Could you check a few things on this model? Use its own coordinates, in mm. Give positions to 0.01 mm unless a question says otherwise; leave off trailing zeros. Write each loop counter-clockwise with the first axis right and the second up, starting at its lowest first coordinate (ties: lowest second). Pieces come first, ordered by that corner, then holes. Notation, with made-up numbers: (-38.5, 48) -> (-18.5, 48) arc R21 ccw to (-18.5, 69) -> close; hole circle Ø2 at (-1.75, -17.5). An arc over 180 degrees is marked (long way). One line per question, with ' | ' between items.
from build123d import *

# Parameters (mm, degrees)
MODEL_R                 = 1.5
SALIENTE_EXTRUIR1_DEPTH = 3


with BuildPart() as part:
    # Model → Saliente-Extruir1 (new body)
    with BuildSketch(Plane.XY):
        with BuildLine():
            Line((-105.943383637, 101.056539338), (-105.943383637, 56.056539338))
            ThreePointArc((-105.943383637, 56.056539338), (-104.625364152, 52.874558823), (-101.443383637, 51.556539338))
            Line((-101.443383637, 51.556539338), (-56.443383637, 51.556539338))
            ThreePointArc((-56.443383637, 51.556539338), (-54.721308191, 51.899081442), (-53.261403122, 52.874558823))
            Line((-53.261403122, 52.874558823), (-104.625364152, 104.238519853))
            ThreePointArc((-104.625364152, 104.238519853), (-105.600841533, 102.778614784), (-105.943383637, 101.056539338))
        make_face()
        with Locations((-101.443383637, 92.056539338)):
            Circle(MODEL_R, mode=Mode.SUBTRACT)
        with Locations((-101.443383637, 83.056539338)):
            Circle(MODEL_R, mode=Mode.SUBTRACT)
        with Locations((-92.443383637, 83.056539338)):
            Circle(MODEL_R, mode=Mode.SUBTRACT)
        with Locations((-101.443383637, 74.056539338)):
            Circle(MODEL_R, mode=Mode.SUBTRACT)
        with Locations((-92.443383637, 74.056539338)):
            Circle(MODEL_R, mode=Mode.SUBTRACT)
        with Locations((-83.443383637, 74.056539338)):
            Circle(MODEL_R, mode=Mode.SUBTRACT)
        with Locations((-101.443383637, 65.056539338)):
            Circle(MODEL_R, mode=Mode.SUBTRACT)
        with Locations((-92.443383637, 65.056539338)):
            Circle(MODEL_R, mode=Mode.SUBTRACT)
        with Locations((-83.443383637, 65.056539338)):
            Circle(MODEL_R, mode=Mode.SUBTRACT)
        with Locations((-74.443383637, 65.056539338)):
            Circle(MODEL_R, mode=Mode.SUBTRACT)
        with Locations((-101.443383637, 56.056539338)):
            Circle(MODEL_R, mode=Mode.SUBTRACT)
        with Locations((-92.443383637, 56.056539338)):
            Circle(MODEL_R, mode=Mode.SUBTRACT)
        with Locations((-83.443383637, 56.056539338)):
            Circle(MODEL_R, mode=Mode.SUBTRACT)
        with Locations((-74.443383637, 56.056539338)):
            Circle(MODEL_R, mode=Mode.SUBTRACT)
        with Locations((-65.443383637, 56.056539338)):
            Circle(MODEL_R, mode=Mode.SUBTRACT)
    extrude(amount=SALIENTE_EXTRUIR1_DEPTH)


solid = part.part
Q1. If I drill on line 1 along X through (y, z) = (55, 2.15); line 2 along Y through (x, z) = (-73.5, 0.25); line 3 along Y through (x, z) = (-100.5, 2.9), over which ranges is the centre line in solid material (lowest first)?
Answer below:
line 1: x = -105.82 to -102.51, -100.38 to -93.51, -91.38 to -84.51, -82.38 to -75.51, -73.38 to -66.51, -64.38 to -55.39 | line 2: y = 51.56 to 54.89, 57.22 to 63.89, 66.22 to 73.11 | line 3: y = 51.56 to 54.89, 57.22 to 63.89, 66.22 to 72.89, 75.22 to 81.89, 84.22 to 90.89, 93.22 to 100.11
Q2. Imagine slicing it at D-D on x = -88. Please give me the cut outline in (y, z).
Answer below:
outline: (51.56, 0) -> (87.61, 0) -> (87.61, 3) -> (51.56, 3) -> close
Q3. Imagine slicing it at A-A on x = -74. Please give me the cut outline in (y, z).
Answer below:
outline: (51.56, 0) -> (54.62, 0) -> (54.62, 3) -> (51.56, 3) -> close; (57.49, 0) -> (63.62, 0) -> (63.62, 3) -> (57.49, 3) -> close; (66.49, 0) -> (73.61, 0) -> (73.61, 3) -> (66.49, 3) -> close
Q4. Imagine slicing it at C-C on x = -81. Please give me the cut outline in (y, z).
Answer below:
outline: (51.56, 0) -> (80.61, 0) -> (80.61, 3) -> (51.56, 3) -> close
Q5. If we mould it in two halves opening along X, with no side actions, what happens to faces 1 (the cylindrical face through (-104.66, 52.91, 1.48)), 2 (the cylindrical face through (-82.8, 63.7, 1.5)), 3 (the cylindrical face through (-91.8, 63.7, 1.5)), 4 (the flat face through (-86, 72, 3))? For each: +X half, -X half, draft (parallel to the pull), parting line (faces both ways), or undercut.
Answer below:
face 1: -X half | face 2: undercut | face 3: undercut | face 4: draft
Q6. Imagine slicing it at B-B on z = 0.6. Count the separate pieces of the cut face and the enclosed holes in it, and give its area (3 significant figures).
Answer below:
separate pieces: 1 | enclosed holes: 15 | area: 1,340 mm^2
